Read the model definition and answer for the solid it produces. Units are mm, in the model's axes. Face numbers are marked on the shaded views. A direction names the side the tool comes from. Give positions to 0.01 mm unless a question says otherwise; leave off trailing zeros. Loops run counter-clockwise (first coordinate to the right, second up) from the corner with the lowest first, then second, coordinate; pieces in that order, holes last.
(1) Find section C-C, the plane y = 8. Write down the section's boundary in (x, z).
(2) Find section B-B, the plane z = -24. Write down the section's boundary in (x, y), then the cut area to 3 significant figures.
(3) Find section D-D, the plane x = 40.5. Write down the section's boundary in (y, z).
(4) Find section A-A, the plane x = 0. Write down the section's boundary in (y, z).
(5) Each of these flat-tipped pins is pushed along its axis until it touches: P1, Ø5, axis at x = 15, y = 3, coming from the +Z side; P2, Ø2, axis at y = 6, z = -27, coming from the +X side; P3, Ø1, axis at x = 12.5, y = 7, coming from the +Z side. Where does it stop, or does it pass through?
(6) Straight lines are drawn through the part: probe 1 along X at (y, z) = (6.5, -30); probe 2 along X at (y, z) = (0.5, 1); probe 3 along X at (y, z) = (12, -23). For each, find the intervals that lie inside material, in ascending order.
(7) Which of the six approach directions +Z, -Z, +X, -X, +Y, -Y give full straight-line access (tool end or side, diameter ignored) to the marked faces 4, 5, 6 and 7?
(8) Determine the mould class of the marked faces 1, 2 and 3 for opening direction X: pulls with the +X half, pulls with the -X half, needs draft (parallel to the pull), parting line crosses it, or undercut.
```python
from build123d import *

# Parameters (mm, degrees)
SKETCH_1_R        = 4.5
SKETCH_1_R_2      = 2.05
EXTRUDE_1_DEPTH   = 15
EXTRUDE_1_2_DEPTH = 15
EXTRUDE_1_3_DEPTH = 15
EXTRUDE_1_4_DEPTH = 15
SKETCH_2_R        = 2.05
EXTRUDE_2_DEPTH   = 15
EXTRUDE_START     = -15
SKETCH_3_R        = 2.05
EXTRUDE_3_DEPTH   = 15
FILLET_1_R        = 1.5


with BuildPart() as part:
    # Sketch 1 → Extrude 1 (new body)
    with BuildSketch(Plane(origin=(0, 0, 0), x_dir=(1, 0, 0), z_dir=(0, 1, 0))):
        with Locations(Location((0, 0, 0), (0, 0, 270))):
            Circle(SKETCH_1_R)
        with Locations(Location((0, 0, 0), (0, 0, 270))):
            Circle(SKETCH_1_R_2, mode=Mode.SUBTRACT)
    extrude(amount=EXTRUDE_1_DEPTH)



with BuildPart() as body_2:
    # Sketch 1 → Extrude 1 2 (new body)
    with BuildSketch(Plane(origin=(0, 0, 0), x_dir=(1, 0, 0), z_dir=(0, 1, 0))):
        with Locations(Location((0, 30, 0), (0, 0, 270))):
            Circle(SKETCH_1_R)
        with Locations(Location((0, 30, 0), (0, 0, 270))):
            Circle(SKETCH_1_R_2, mode=Mode.SUBTRACT)
    extrude(amount=EXTRUDE_1_2_DEPTH)



with BuildPart() as body_3:
    # Sketch 1 → Extrude 1 3 (new body)
    with BuildSketch(Plane(origin=(0, 0, 0), x_dir=(1, 0, 0), z_dir=(0, 1, 0))):
        with Locations(Location((50, 30, 0), (0, 0, 270))):
            Circle(SKETCH_1_R)
        with Locations(Location((50, 30, 0), (0, 0, 270))):
            Circle(SKETCH_1_R_2, mode=Mode.SUBTRACT)
    extrude(amount=EXTRUDE_1_3_DEPTH)


with BuildPart() as body_4:
    # Sketch 1 → Extrude 1 4 (new body)
    with BuildSketch(Plane(origin=(0, 0, 0), x_dir=(1, 0, 0), z_dir=(0, 1, 0))):
        with Locations(Location((50, 0, 0), (0, 0, 270))):
            Circle(SKETCH_1_R)
        with Locations(Location((50, 0, 0), (0, 0, 270))):
            Circle(SKETCH_1_R_2, mode=Mode.SUBTRACT)
    extrude(amount=EXTRUDE_1_4_DEPTH)


with BuildPart() as body_2_1:
    add(body_2.part)

    add(body_4.part)  # Extrude 2 merges body 4
    # Sketch 2 → Extrude 2 (add)
    with BuildSketch(Plane(origin=(0, 15, 0), x_dir=(1, 0, 0), z_dir=(0, 1, 0))):
        with BuildLine():
            Line((51.543487266, 2.572478777), (1.543487266, 32.572478777))
            ThreePointArc((1.543487266, 32.572478777), (-2.572478777, 31.543487266), (-1.543487266, 27.427521223))
            Line((-1.543487266, 27.427521223), (48.456512734, -2.572478777))
            ThreePointArc((48.456512734, -2.572478777), (52.572478777, -1.543487266), (51.543487266, 2.572478777))
        make_face()
        with Locations(Location((0, 30, 0), (0, 0, 270))):
            Circle(SKETCH_2_R, mode=Mode.SUBTRACT)
        with Locations(Location((50, 0, 0), (0, 0, 270))):
            Circle(SKETCH_2_R, mode=Mode.SUBTRACT)
    extrude(amount=-EXTRUDE_2_DEPTH)


with BuildPart() as part_1:
    add(part.part)

    add(body_2_1.part)  # Extrude 3 merges body 2

    add(body_3.part)  # Extrude 3 merges body 3
    # Sketch 3 → Extrude 3 (add)
    with BuildSketch(Plane(origin=(0, 15, 0), x_dir=(1, 0, 0), z_dir=(0, 1, 0)).offset(EXTRUDE_START)):
        with BuildLine():
            Line((-1.543487266, 2.572478777), (48.456512734, 32.572478777))
            ThreePointArc((48.456512734, 32.572478777), (52.572478777, 31.543487266), (51.543487266, 27.427521223))
            Line((51.543487266, 27.427521223), (1.543487266, -2.572478777))
            ThreePointArc((1.543487266, -2.572478777), (-2.572478777, -1.543487266), (-1.543487266, 2.572478777))
        make_face()
        with Locations(Location((0, 0, 0), (0, 0, 270))):
            Circle(SKETCH_3_R, mode=Mode.SUBTRACT)
        with Locations(Location((50, 30, 0), (0, 0, 270))):
            Circle(SKETCH_3_R, mode=Mode.SUBTRACT)
    extrude(amount=EXTRUDE_3_DEPTH)

    # Fillet 1
    fillet_1_edges = [part_1.edges().sort_by_distance(p)[0] for p in [
        (1.332631442, 7.5, -4.298150002),
        (4.419605974, 7.5, 0.846807552),
        (45.580394026, 7.5, -30.846807552),
        (48.667368558, 7.5, -25.701849998),
        (30.830951895, 7.5, -15),
        (48.667368558, 7.5, -4.298150002),
        (25, 7.5, -11.501428863),
        (45.580394026, 7.5, 0.846807552),
        (25, 7.5, -18.498571137),
        (19.169048105, 7.5, -15),
        (4.419605974, 7.5, -30.846807552),
        (1.332631442, 7.5, -25.701849998),
    ]]
    fillet(fillet_1_edges, radius=FILLET_1_R)


solid = part_1.part
```
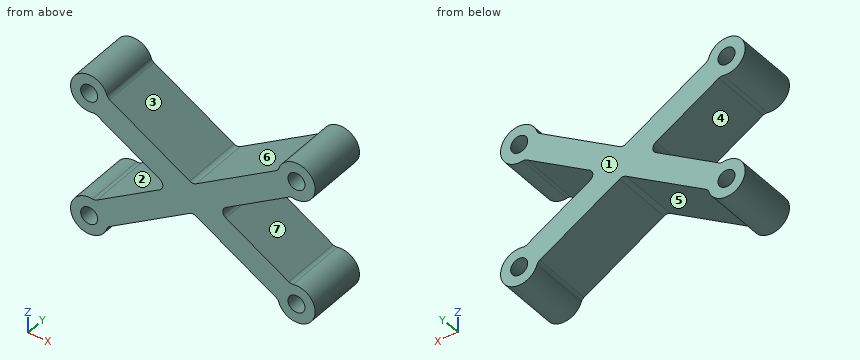
Entries:
1. outline: (0.82, -25.57) arc R4.5 ccw (long way) to (4.29, -31.36) arc R1.5 cw to (4.95, -30.53) - (24.23, -18.96) arc R1.5 cw to (25.77, -18.96) - (45.05, -30.53) arc R1.5 cw to (45.71, -31.36) arc R4.5 ccw (long way) to (49.18, -25.57) arc R1.5 cw to (48.14, -25.39) - (32.97, -16.29) arc R1.5 cw to (32.97, -13.71) - (48.14, -4.61) arc R1.5 cw to (49.18, -4.43) arc R4.5 ccw (long way) to (45.71, 1.36) arc R1.5 cw to (45.05, 0.53) - (25.77, -11.04) arc R1.5 cw to (24.23, -11.04) - (4.95, 0.53) arc R1.5 cw to (4.29, 1.36) arc R4.5 ccw (long way) to (0.82, -4.43) arc R1.5 cw to (1.86, -4.61) - (17.03, -13.71) arc R1.5 cw to (17.03, -16.29) - (1.86, -25.39) arc R1.5 cw to start; hole circle Ø4.1 at (0, -30); hole circle Ø4.1 at (0, 0); hole circle Ø4.1 at (50, -30); hole circle Ø4.1 at (50, 0)
2. outline: (4.17, 0) - (15.83, 0) - (15.83, 15) - (4.17, 15) - close; (34.17, 0) - (45.83, 0) - (45.83, 15) - (34.17, 15) - close
2. area: 350 mm2
3. outline: (0, -27.8) - (15, -27.8) - (15, -20.8) - (0, -20.8) - close; (0, -9.2) - (15, -9.2) - (15, -2.2) - (0, -2.2) - close
4. outline: (0, -34.5) - (15, -34.5) - (15, -32.05) - (0, -32.05) - close; (0, -27.95) - (15, -27.95) - (15, -25.5) - (0, -25.5) - close; (0, -4.5) - (15, -4.5) - (15, -2.05) - (0, -2.05) - close; (0, 2.05) - (15, 2.05) - (15, 4.5) - (0, 4.5) - close
5. P1: stops at z = -4
5. P2: stops at x = 54.03
5. P3: stops at z = -3.7
6. probe 1: x = -4.5 to -2.05, 2.05 to 5.83, 44.17 to 47.95, 52.05 to 54.5
6. probe 2: x = -4.39 to -1.79, 1.79 to 4.46, 45.54 to 48.21, 51.79 to 54.39
6. probe 3: x = 5.84 to 17.5, 32.5 to 44.16
7. face 4: -X, +Y, -Y
7. face 5: -Z, +Y, -Y
7. face 6: +Z, +Y, -Y
7. face 7: +X, +Y, -Y
8. face 1: needs draft
8. face 2: pulls with the -X half
8. face 3: undercut
